Can you work these out from the model? Positions are in its coordinate system, mm. A direction names the side the tool comes from. Give positions to 0.01 mm unless a question says otherwise; leave off trailing zeros. Loops run counter-clockwise (first coordinate to the right, second up) from the corner with the lowest first, then second, coordinate; pieces in that order, holes last. Notation, with made-up numbers: (-5.75, 14.25) -> (32.25, 14.25) arc R23 ccw to (32.25, 32.25) -> close; hole circle Ø8 at (43.25, 35). An arc over 180 degrees is marked (long way). Use CSV: the item, a comma, the result in double quotes.
Autodesk Inventor part; units mm, degrees
ref_plane "YZ Plane" through (0, 0, 0) normal (1, 0, 0) x (0, 1, 0)
ref_plane "XZ Plane" through (0, 0, 0) normal (0, 1, 0) x (-1, 0, 0)
ref_plane "XY Plane" through (0, 0, 0) normal (0, 0, 1) x (1, 0, 0)
sketch "草圖1" plane through (0, 0, 0) normal (0, 1, 0) x (-1, 0, 0)
  line L0 (10, 15) -> (-10, 15)
  line L1 (-10, 15) -> (-10, -5)
  line L2 (-10, -15) -> (10, -15) construction
  line L3 (10, -15) -> (10, -5) construction
  arc A0 (-10, -5) -> (10, -5) centre (0, -5) ccw
  line L4 (10, -5) -> (10, 15)
  line L5 (-10, -5) -> (-10, -15) construction
  circle A1 centre (0, -5) radius 5
  point P0 (0, 0)
  point P1 (10, 0)
  point P2 (0, 15)
  dimension "d0" = 30
  dimension "d1" = 20
  dimension "d2" = 5
  dimension "d3" = 10
extrude "擠出1" add sketch "草圖1" along normal blind 5
sketch "草圖2" plane through (-10, 0, 15) normal (0, 0, 1) x (1, 0, 0)
  line L0 (0, 0) -> (20, 0) construction
  line L1 (20, 0) -> (20, 5) construction
  line L2 (0, 5) -> (20, 5) construction
  line L3 (0, 0) -> (0, 5) construction
  line L4 (0, 5) -> (20, 5)
  line L5 (0, 5) -> (20, 5)
  line L6 (20, 5) -> (20, 10)
  line L7 (0, 10) -> (0, 5)
  arc A0 (20, 10) -> (0, 10) centre (10, 10) ccw
  circle A1 centre (10, 10) radius 5
  point P0 (10, 0)
  dimension "d6" = 5
  dimension "d7" = 10
  dimension "d8" = 10
extrude "擠出2" add sketch "草圖2" against normal blind 5
sketch "草圖3" plane through (-10, 0, 10) normal (0, 0, -1) x (-1, 0, 0)
  line L0 (-10, 5) -> (-20, 5)
  circle A0 centre (-10, 10) radius 5
  line L1 (0, 5) -> (-10, 5)
  line L2 (0, 5) -> (0, 10)
  arc A1 (0, 10) -> (-20, 10) centre (-10, 10) ccw
  line L3 (-20, 10) -> (-20, 5)
  line L4 (-20, 10) -> (-20, 5)
  line L5 (0, 5) -> (0, 10)
  line L6 (-20, 5) -> (0, 5)
  line L7 (0, 5) -> (0, 10)
  line L8 (0, 10) -> (-5, 10)
  line L9 (-20, 10) -> (-20, 5)
  line L10 (-15, 10) -> (-20, 10)
  line L11 (-5, 10) -> (-15, 10) construction
  point P0 (-10, 0)
  dimension "d11" = 5
extrude "擠出3" add sketch "草圖3" along normal blind 5 contours L0 L3 L10 A0 | A0 L8 L2 L1
properties part number "8"
(1) Will these pins go through, and if not, where does the flat tip stop? pin 1 Ø4 at (x, z) = (8, 7.5) entering from +Y; pin 2 Ø2 at (x, y) = (6, 7.5) entering from -Z; pin 3 Ø5.5 at (x, y) = (6.5, 6.5) entering from -Z.
Answer sheet:
pin 1,"stops at y = 10"
pin 2,"stops at z = 5"
pin 3,"stops at z = -14.08"
(2) If I drill on L1, parallel to Z at x = 0.25, y = 2; L2, parallel to X at y = 10, z = 11.5; L3, parallel to Y at x = 0, z = 12.75, over which ranges is the centre line in solid material (lowest first)? Write a range as from..to.
Answer sheet:
L1,"z = -15..-9.99, -0.01..15"
L2,"x = -10..-5, 5..10"
L3,"y = 0..5, 15..20"
(3) Which directions (+Z, -Z, +X, -X, +Y, -Y) give clear straight access to the entire face, cutting with the end or side of a thin tool? Please do faces 1 (the face through (7, 10, 8)), 2 (the face through (0, 2, -15)).
Answer sheet:
face 1,"-Z, +X, -X, +Y"
face 2,"-Z, +Y, -Y"
(4) If we section it at C-C, the plane y = 6.75: Write out the boundary of the cut face in (x, z), then the cut area to 3 significant figures.
Answer sheet:
outline,"(-10, 5) -> (-3.8, 5) -> (-3.8, 15) -> (-10, 15) -> close; (3.8, 5) -> (10, 5) -> (10, 15) -> (3.8, 15) -> close"
area,"124 mm2"
(5) If we section it at A-A, the plane x = -2.75: Write out the boundary of the cut face in (y, z), then the cut area to 3 significant figures.
Answer sheet:
outline,"(0, -14.61) -> (5, -14.61) -> (5, -9.18) -> (0, -9.18) -> close; (0, -0.82) -> (5, -0.82) -> (5, 5) -> (5.82, 5) -> (5.82, 15) -> (0, 15) -> close; (14.18, 10) -> (19.61, 10) -> (19.61, 15) -> (14.18, 15) -> close"
area,"142 mm2"
(6) If we section it at D-D, the plane z = 3: Write out the boundary of the cut face in (x, y), then the cut area to 3 significant figures.
Answer sheet:
outline,"(-10, 0) -> (10, 0) -> (10, 5) -> (-10, 5) -> close"
area,"100 mm2"
(7) We'd pull the mould along X, two halves only. Please class faces 3 (the face through (-8, 10, 8)), 4 (the face through (10, 4, 7)), 5 (the face through (2.307, 5.564, 11.181)), 6 (the face through (1.08, 2.46, -0.12)): released by +X, released by -X, zero draft, split by the parting line, or undercut.
Answer sheet:
face 3,"zero draft"
face 4,"released by +X"
face 5,"undercut"
face 6,"undercut"
(8) If we section it at B-B, the plane z = -2.75: Write out the boundary of the cut face in (x, y).
Answer sheet:
outline,"(-10, 0) -> (-4.47, 0) -> (-4.47, 5) -> (-10, 5) -> close; (4.47, 0) -> (10, 0) -> (10, 5) -> (4.47, 5) -> close"
